Read the model definition and answer for the solid it produces. Units are mm, in the model's axes. Face numbers are marked on the shaded views. A direction names the side the tool comes from. Coordinates: 2 decimals unless noted, no trailing zeros. Loops run counter-clockwise (first coordinate to the right, second up) from the corner with the lowest first, then second, coordinate; pieces in that order, holes last. Notation, with made-up numbers: (15.5, 61.5) - (45.5, 61.5) arc R23 ccw to (45.5, 81.5) - close; hole circle Ø7 at (41.25, 20.5). An arc over 180 degrees is marked (long way). Use one line per item in the form item = value.
from build123d import *

# Parameters (mm, degrees)
SKICA1_W                 = 240
SKICA1_H                 = 69
SKICA1_W_2               = 226
SKICA1_H_2               = 57
P_IDAT_VYSUNUT_M1_DEPTH  = 50.7
SKICA2_R                 = 13.1
ODEBRAT_VYSUNUT_M1_DEPTH = 3
SKICA4_R                 = 10.6
ODEBRAT_VYSUNUT_M2_DEPTH = 6
P_IDAT_VYSUNUT_M2_DEPTH  = 6


with BuildPart() as part:
    # Skica1 → Přidat vysunutím1 (new body)
    with BuildSketch(Plane(origin=(0, 0, 0), x_dir=(1, 0, 0), z_dir=(0, 1, 0))):
        with Locations((120, 34.5)):
            Rectangle(SKICA1_W, SKICA1_H)
        with Locations((120, 34.5)):
            Rectangle(SKICA1_W_2, SKICA1_H_2, mode=Mode.SUBTRACT)
    extrude(amount=P_IDAT_VYSUNUT_M1_DEPTH)

    # Skica2 → Odebrat vysunutím1 (cut)
    with BuildSketch(Plane.XY):
        with Locations((46.25, 35.6)):
            Circle(SKICA2_R)
        with Locations((73.75, 35.6)):
            Circle(SKICA2_R)
        with Locations((101.25, 35.6)):
            Circle(SKICA2_R)
        with Locations((138.75, 35.6)):
            Circle(SKICA2_R)
        with Locations((166.25, 35.6)):
            Circle(SKICA2_R)
        with Locations((193.75, 35.6)):
            Circle(SKICA2_R)
        with Locations((120, 15.1)):
            Circle(SKICA2_R)
    extrude(amount=-ODEBRAT_VYSUNUT_M1_DEPTH, mode=Mode.SUBTRACT)

    # Skica4 → Odebrat vysunutím2 (cut)
    with BuildSketch(Plane.XY):
        with Locations((46.25, 35.6)):
            Circle(SKICA4_R)
        with Locations((73.75, 35.6)):
            Circle(SKICA4_R)
        with Locations((138.75, 35.6)):
            Circle(SKICA4_R)
        with Locations((101.25, 35.6)):
            Circle(SKICA4_R)
        with Locations((120, 15.1)):
            Circle(SKICA4_R)
        with Locations((166.25, 35.6)):
            Circle(SKICA4_R)
        with Locations((193.75, 35.6)):
            Circle(SKICA4_R)
    extrude(amount=-ODEBRAT_VYSUNUT_M2_DEPTH, mode=Mode.SUBTRACT)

    # Skica5 → Přidat vysunutím2 (add)
    with BuildSketch(Plane.XZ):
        Polygon((149.130434783, -6), (129.075362319, -6), (233, -38.594545455), (233, -32.304545455), align=None)
        Polygon((90.869565217, -6), (7, -32.304545455), (7, -38.594545455), (110.924637681, -6), align=None)
    extrude(amount=-P_IDAT_VYSUNUT_M2_DEPTH)


solid = part.part
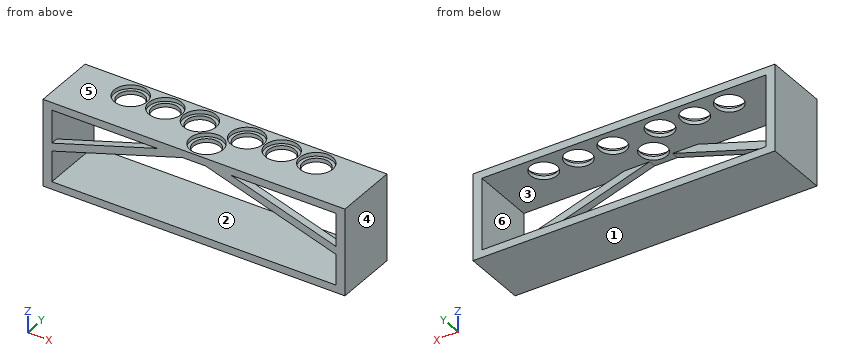
Item 1: For a pull along X with two mould halves and no side action, classify the marked faces 3, 4, 5 and 6 as +X half, -X half, draft (parallel to the pull), parting line (faces both ways), or undercut.
Results below:
face_3 = undercut
face_4 = +X half
face_5 = draft
face_6 = undercut
Item 2: The part is cut by section D-D on y = 9. Give the vertices of the cut face in (x, z), plus the area to 3 significant figures.
Results below:
outline = (0, -69) - (240, -69) - (240, 0) - (131.59, 0) - (131.59, -3) - (128.67, -3) - (128.67, -6) - (233, -6) - (233, -63) - (7, -63) - (7, -6) - (111.33, -6) - (111.33, -3) - (108.41, -3) - (108.41, 0) - (0, 0) - close
area = 3,560 mm²
Item 3: The part is cut by section B-B on z = -10. Give the vertices of the cut face in (x, y).
Results below:
outline = (0, 0) - (7, 0) - (7, 50.7) - (0, 50.7) - close; (78.12, 0) - (98.17, 0) - (98.17, 6) - (78.12, 6) - close; (141.83, 0) - (161.88, 0) - (161.88, 6) - (141.83, 6) - close; (233, 0) - (240, 0) - (240, 50.7) - (233, 50.7) - close
Item 4: Which of the six approach directions +Z, -Z, +X, -X, +Y, -Y give full straight-line access (tool end or side, diameter ignored) to the marked faces 1 and 2?
Results below:
face_1 = -Z, +X, -X, +Y, -Y
face_2 = +Y, -Y
Item 5: Each of these flat-tipped pins is pushed along its axis until it touches: P1, Ø23.5, axis at x = 101.25, y = 35.6, coming from the +Z side; P2, Ø13, axis at x = 50, y = 34.5, coming from the +Z side; P3, Ø1, axis at x = 156.5, y = 17.5, coming from the +Z side; P4, Ø10, axis at x = 78.5, z = -18, coming from the +Y side. Where does it stop, or does it pass through?
Results below:
P1 = -3
P2 = -63
P3 = 0
P4 = 6
Item 6: The part is cut by section A-A on x = 120. Give the vertices of the cut face in (y, z), plus the area to 3 significant figures.
Results below:
outline = (0, -69) - (50.7, -69) - (50.7, -63) - (0, -63) - close; (0, -6) - (4.5, -6) - (4.5, -3) - (2, -3) - (2, 0) - (0, 0) - close; (25.7, -6) - (50.7, -6) - (50.7, 0) - (28.2, 0) - (28.2, -3) - (25.7, -3) - close
area = 466 mm²
Item 7: Find the intervals of material crossed by L1, parallel to Y at x = 73.75, z = -1; L2, parallel to Z at x = 203, y = 30; L3, parallel to X at y = 49, z = -22, in increasing order.
Results below:
L1 = 0 to 22.5, 48.7 to 50.7
L2 = -69 to -63, -6 to -3
L3 = 0 to 7, 233 to 240
Item 8: The part is cut by section C-C on x = 166.25. Give the vertices of the cut face in (y, z).
Results below:
outline = (0, -69) - (50.7, -69) - (50.7, -63) - (0, -63) - close; (0, -17.66) - (6, -17.66) - (6, -11.37) - (0, -11.37) - close; (0, -6) - (25, -6) - (25, -3) - (22.5, -3) - (22.5, 0) - (0, 0) - close; (46.2, -6) - (50.7, -6) - (50.7, 0) - (48.7, 0) - (48.7, -3) - (46.2, -3) - close
